Source: CAD feature listing. Evaluate the final solid. Frame: model axes, mm. A direction names the side the tool comes from. Coordinates: 2 decimals unless noted, no trailing zeros. Order: outer loops, then holes, each group sorted by start corner. A loop starts at its lowest first (then second) coordinate and runs counter-clockwise, first axis right, second up. Notation, with made-up numbers: (-2.5, 48.25) - (56.5, 48.25) arc R25 ccw to (56.5, 65.25) - close; hole circle Ø8 at (83.5, -16.5). An arc over 180 degrees is marked (long way). One line per question, with ' | ' between items.
from build123d import *

# Parameters (mm, degrees)
F0_R      = 7.493
F1_DEPTH  = 75.184
F2_R      = 5.08
F3_DEPTH  = 12.7
F4_R      = 5.08
F5_DEPTH  = 11.684
F8_R      = 2.921
F9_DEPTH  = 82.55
F10_R     = 2.38125
F11_DEPTH = 19.05


with BuildPart() as f1:
    # F0 (on Front) → F1 (new body)
    with BuildSketch(Plane.XZ):
        Circle(F0_R)
    extrude(amount=F1_DEPTH)

    # F2 (on face) → F3 (join)
    with BuildSketch(Plane(origin=(0, 0, 0), x_dir=(-1, 0, 0), z_dir=(0, 1, 0))):
        Circle(F2_R)
    extrude(amount=F3_DEPTH)

    # F4 (on face) → F5 (join)
    with BuildSketch(Plane.XZ.offset(75.184)):
        Circle(F4_R)
    extrude(amount=F5_DEPTH)

    # F6 (on Right) → F7 (revolve)
    with BuildSketch(Plane.YZ):
        with BuildLine():
            ThreePointArc((19.812, -7.366), (25.0205485502, -5.2085485502), (27.178, 0))
            ThreePointArc((27.178, 0), (25.0205485502, 5.2085485502), (19.812, 7.366))
            Line((19.812, 7.366), (19.812, 0))
            Line((19.812, 0), (19.812, -7.366))
        make_face()
    revolve(axis=Axis((0, 19.812, 3.683), (0, 0, 1)))

    # F8 (on face) → F9 (cut)
    with BuildSketch(Plane.XZ.offset(86.868)):
        Circle(F8_R)
    extrude(amount=-F9_DEPTH, mode=Mode.SUBTRACT)

    # F10 (on Right) → F11 (join)
    with BuildSketch(Plane.YZ):
        with Locations((19.812, 0)):
            Circle(F10_R)
    extrude(amount=F11_DEPTH)


solid = f1.part
(1) Material intervals for L1, parallel to Z at x = 0, y = -24; L2, parallel to Y at x = 4.5, z = 1.25; L3, parallel to Y at x = 6.25, z = -1.75, sorted ascending. Write a range as from..to.
Taken from the geometry:
L1: z = -7.49..-2.92, 2.92..7.49 | L2: y = -86.87..12.7, 14.12..25.51 | L3: y = -75.18..0, 16.33..23.3
(2) Pin query (flat end, axial travel): P1, Ø5, axis at y = -45.5, z = -0.5, coming from the +X side; P2, Ø3, axis at x = 1, z = -2, coming from the +Y side; P3, Ø6, axis at x = 13.5, z = -5, coming from the +Y side. Return the tip coordinate at first contact, or that it passes through.
Taken from the geometry:
P1: stops at x = 7.49 | P2: stops at y = 27.14 | P3: stops at y = 21.1
(3) Pull-direction query (X, two-part tool) for faces 1 (the flat face through (2.2, -86.868, -2.2)), 2 (the flat face through (0, -4.318, 0)), 3 (the flat face through (19.05, 20, 0)), 4 (the cylindrical face through (-0.98, -37.07, 7.43)); classes: pulls with the +X half, pulls with the -X half, needs draft (parallel to the pull), parting line crosses it, or undercut.
Taken from the geometry:
face 1: needs draft | face 2: undercut | face 3: pulls with the +X half | face 4: parting line crosses it
(4) Cut plane B-B (x = 0). Return the cut outline in (y, z).
Taken from the geometry:
outline: (-86.87, -5.08) - (-75.18, -5.08) - (-75.18, -7.49) - (0, -7.49) - (0, -5.08) - (12.7, -5.08) - (12.7, -1.92) arc R7.37 ccw (long way) to (12.7, 1.92) - (12.7, 5.08) - (0, 5.08) - (0, 7.49) - (-75.18, 7.49) - (-75.18, 5.08) - (-86.87, 5.08) - (-86.87, 2.92) - (-4.32, 2.92) - (-4.32, -2.92) - (-86.87, -2.92) - close
(5) Set-up query: faces 5 (the cylindrical face through (-0.661, -80.944, 5.037)), 6 (the flat face through (5, 0, -2)), 7 (the cylindrical face through (12.926, 17.433, 0.105)). Return all of +Z, -Z, +X, -X, +Y, -Y with unobstructed straight access to the full face (end or side cutting, diameter ignored); none if empty.
Taken from the geometry:
face 5: -Y | face 6: none | face 7: +X
(6) Cut plane C-C (y = 1). Return the cut outline in (x, z), and give its area (3 significant figures).
Taken from the geometry:
outline: circle Ø10.16 at (0, 0) | area: 81.1 mm²
(7) Cut plane A-A (z = 6.25). Return the cut outline in (x, y).
Taken from the geometry:
outline: (-4.13, -75.18) - (4.13, -75.18) - (4.13, 0) - (-4.13, 0) - close; circle Ø7.8 at (0, 19.81)
